CAD build for the part. Positions are in the model's coordinates, mm. Face numbers are marked on the shaded views. A direction names the side the tool comes from. Give positions to 0.01 mm unless a question says otherwise; leave off trailing zeros. Loops run counter-clockwise (first coordinate to the right, second up) from the corner with the lowest first, then second, coordinate; pieces in that order, holes last.
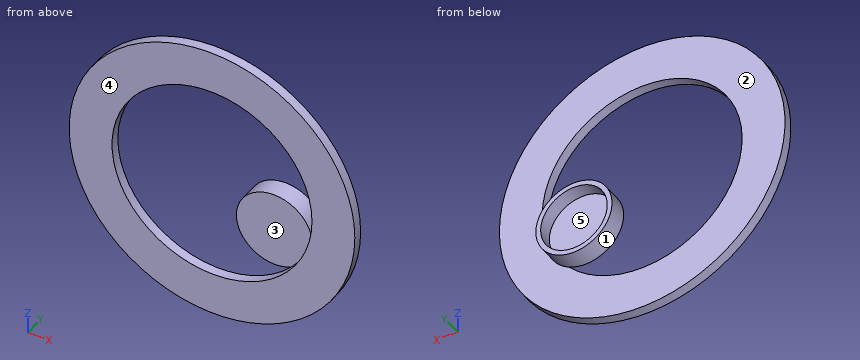
```python
from build123d import *

# Parameters (mm, degrees)
SKETCH1_R           = 30
BOSS_EXTRUDE1_DEPTH = 2
SKETCH2_R           = 21
CUT_EXTRUDE1_DEPTH  = 2
SKETCH3_R           = 8
BOSS_EXTRUDE2_DEPTH = 4
SKETCH4_R           = 7
CUT_EXTRUDE2_DEPTH  = 3


with BuildPart() as part:
    # Sketch1 → Boss-Extrude1 (new body)
    with BuildSketch(Plane(origin=(0, 0, 0), x_dir=(1, 0, 0), z_dir=(0, 1, 0))):
        Circle(SKETCH1_R)
    extrude(amount=BOSS_EXTRUDE1_DEPTH)

    # Sketch2 → Cut-Extrude1 (cut)
    with BuildSketch(Plane(origin=(0, 2, 0), x_dir=(1, 0, 0), z_dir=(0, 1, 0))):
        Circle(SKETCH2_R)
    extrude(amount=-CUT_EXTRUDE1_DEPTH, mode=Mode.SUBTRACT)

    # Sketch3 → Boss-Extrude2 (add)
    with BuildSketch(Plane(origin=(0, 2, 0), x_dir=(1, 0, 0), z_dir=(0, 1, 0))):
        with Locations((11.890730665, 7.098367026)):
            Circle(SKETCH3_R)
    extrude(amount=BOSS_EXTRUDE2_DEPTH)

    # Sketch4 → Cut-Extrude2 (cut)
    with BuildSketch(Plane(origin=(0, 6, 0), x_dir=(1, 0, 0), z_dir=(0, 1, 0))):
        with Locations((11.890730665, 7.098367026)):
            Circle(SKETCH4_R)
    extrude(amount=-CUT_EXTRUDE2_DEPTH, mode=Mode.SUBTRACT)


solid = part.part
```
1. Probe line 1 along X through (y, z) = (0.7, 0); line 2 along X through (y, z) = (4.5, -7.5); line 3 along Y through (x, z) = (-19.5, 15). List the from-to ranges inside material, lowest first.
Responses:
line 1: x = -30 to -21, 21 to 30
line 2: x = 3.9 to 4.9, 18.88 to 19.88
line 3: y = 0 to 2
2. Saw through at C-C, the plane y = 1.15. List the corners of the cut face in (x, z), and give its area (3 significant figures).
Responses:
outline: circle Ø60 at (0, 0); hole circle Ø42 at (0, 0)
area: 1,440 mm2
3. Tool access for the marked faces 4 and 5: list every direction of +Z, -Z, +X, -X, +Y, -Y with a clear straight run to the whole face (end or side of a thin tool).
Responses:
face 4: +Z, -Z, +X, -X, -Y
face 5: +Y
4. Saw through at B-B, the plane z = 3. List the corners of the cut face in (x, y).
Responses:
outline: (-29.85, 0) - (-20.78, 0) - (-20.78, 2) - (-29.85, 2) - close; (20.78, 0) - (29.85, 0) - (29.85, 2) - (20.78, 2) - close
5. Saw through at D-D, the plane z = 24. List the corners of the cut face in (x, y).
Responses:
outline: (-18, 0) - (18, 0) - (18, 2) - (-18, 2) - close
6. Pull direction Z, two halves, no side cores. Call the marked faces 1, 2 and 3: released by +Z, released by -Z, zero draft, split by the parting line, or undercut.
Responses:
face 1: split by the parting line
face 2: zero draft
face 3: undercut
7. Drop flat-ended pins along their axis: pin 1 (3 mm diameter, centred on x = 3, y = 2.5, fed in from -Z); pin 2 (1.5 mm diameter, centred on x = 19, z = -2.5, fed in from -Y); pin 3 (4 mm diameter, centred on x = 12.5, z = 18.5, fed in from +Y). Give the stop position or say it passes through.
Responses:
pin 1: stops at z = -29.96
pin 2: stops at y = 2
pin 3: stops at y = 2
8. Saw through at A-A, the plane x = 0. List the corners of the cut face in (y, z).
Responses:
outline: (0, -30) - (2, -30) - (2, -21) - (0, -21) - close; (0, 21) - (2, 21) - (2, 30) - (0, 30) - close
